Work out the finished part from the listing and answer in its coordinate system (mm). A direction names the side the tool comes from. Give positions to 0.01 mm unless a question says otherwise; leave off trailing zeros. Loops run counter-clockwise (first coordinate to the right, second up) from the corner with the lowest first, then second, coordinate; pieces in that order, holes last. Notation, with made-up numbers: (-25.75, 39.5) - (11.25, 39.5) arc R13 ccw to (11.25, 51.5) - close; hole circle Ø7 at (-10, 5.25). An arc over 180 degrees is marked (long way). Use one line per item in the form item = value. Start each with the question number.
from build123d import *

# Parameters (mm, degrees)
SKETCH1_W           = 20
SKETCH1_H           = 5
BOSS_EXTRUDE1_DEPTH = 30
SKETCH2_W           = 40
SKETCH2_H           = 40
BOSS_EXTRUDE2_DEPTH = 20
FILLET1_R           = 10


with BuildPart() as part:
    # Sketch1 → Boss-Extrude1 (new body)
    with BuildSketch(Plane.XY):
        with Locations((-20, -2.5)):
            Rectangle(SKETCH1_W, SKETCH1_H)
    extrude(amount=BOSS_EXTRUDE1_DEPTH)

    # Sketch2 → Boss-Extrude2 (add)
    with BuildSketch(Plane.XY):
        with Locations((-10, 15)):
            Rectangle(SKETCH2_W, SKETCH2_H)
    extrude(amount=-BOSS_EXTRUDE2_DEPTH)

    # Fillet1
    # the kernel refuses this fillet: 10 mm, written as the material it adds along each edge
    with BuildSketch(Plane(origin=(-10, 0, 0), x_dir=(0, 1, 0), z_dir=(-1, 0, 0))) as fillet1_piece_1:
        with BuildLine():
            CenterArc((FILLET1_R, -FILLET1_R), FILLET1_R, 90, 90)
            Line((0, -FILLET1_R), (0, 0))
            Line((0, 0), (FILLET1_R, 0))
        make_face()
    extrude(amount=20)
    # the kernel refuses this fillet: 10 mm, written as the material it takes off along each edge
    with BuildSketch(Plane(origin=(10, 35, 25), x_dir=(-1, 0, 0), z_dir=(0, 0, -1))) as fillet1_2_piece_1:
        with BuildLine():
            CenterArc((FILLET1_R, -FILLET1_R), FILLET1_R, 90, 90)
            Line((0, -FILLET1_R), (0, 0))
            Line((0, 0), (FILLET1_R, 0))
        make_face()
    extrude(amount=70, mode=Mode.SUBTRACT)
    with BuildSketch(Plane(origin=(11.650635095, 0, 30), x_dir=(0, 0, -1), z_dir=(-1, 0, 0))) as fillet1_2_piece_2:
        with BuildLine():
            CenterArc((8.660254038, 10), FILLET1_R, 210, 60)
            Line((0, 5), (0, 0))
            Line((0, 0), (8.660254038, 0))
        make_face()
    extrude(amount=63.301270189, mode=Mode.SUBTRACT)


solid = part.part
1) A cutting plane is placed at A-A (x = -24). Give the vertices of the cut face in (y, z).
2) A tool of negligible diameter and unlimited length cuts with its end or side. For faces 1 (the flat face through (-20, 0, 16)), 2 (the flat face through (-10, 20, 0)), 3 (the flat face through (-10, -2, 13)), 4 (the flat face through (10, 10, -10)), from which of +Z, -Z, +X, -X, +Y, -Y can it reach the whole face along a straight path? Write none if from no direction.
3) A cutting plane is placed at B-B (y = 13). Give the vertices of the cut face in (x, z).
4) Find the intervals of material crossed by probe 1 along Z at (x, y) = (-7, 23); probe 2 along Y at (x, z) = (0.5, -6); probe 3 along X at (y, z) = (4, 1.5), in increasing order.
5) A cutting plane is placed at C-C (z = 7). Give the vertices of the cut face in (x, y), plus the area to 3 significant figures.
6) Flat-ended cylindrical pins translate along their axes: pin 1 Ø12 at (x, z) = (0, 5) entering from +Y; pin 2 Ø16.5 at (y, z) = (4, 9.5) entering from +X; pin 3 Ø12 at (x, y) = (-10.5, 24.5) entering from +Z; pin 4 Ø5.5 at (x, z) = (-24, 14) entering from +Y. Find the tip coordinate at first contact, or state that the pin passes through.
Answer sheet:
q1.outline = (-5, -20) - (35, -20) - (35, 0) - (10, 0) arc R10 cw to (0, 10) - (0, 21.34) arc R10 ccw to (-5, 30) - close
q2.face_1 = +Z, +X, -X, +Y
q2.face_2 = +Z, +X, +Y
q2.face_3 = +Z, +X, +Y, -Y
q2.face_4 = +Z, -Z, +X, +Y, -Y
q3.outline = (-30, -20) - (10, -20) - (10, 0) - (-30, 0) - close
q4.probe_1 = -20 to 0
q4.probe_2 = -5 to 34.99
q4.probe_3 = -30 to -10
q5.outline = (-30, -5) - (-10, -5) - (-10, 0.46) - (-30, 0.46) - close
q5.area = 109 mm²
q6.pin_1 = 35
q6.pin_2 = -10
q6.pin_3 = 0
q6.pin_4 = 0
